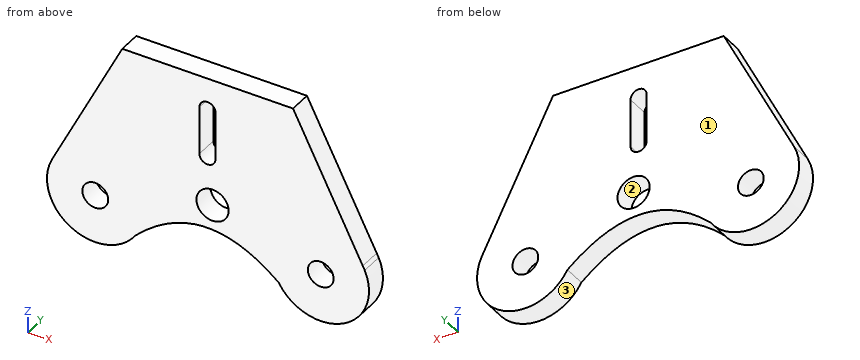
```python
from build123d import *

# Parameters (mm, degrees)
BOSS_EXTRUDE1_DEPTH = 8.89
CUT_EXTRUDE1_DEPTH  = 8.89
SKETCH3_R           = 5.08
CUT_EXTRUDE2_DEPTH  = 8.89
SKETCH4_R           = 5.08
CUT_EXTRUDE3_DEPTH  = 8.89
SKETCH5_R           = 6.35
CUT_EXTRUDE4_DEPTH  = 8.89


with BuildPart() as part:
    # Sketch1 → Boss-Extrude1 (new body)
    with BuildSketch(Plane(origin=(0, 0, 0), x_dir=(1, 0, 0), z_dir=(0, 1, 0))):
        with BuildLine():
            Line((-17.012597889, -8.571698377), (10.66270702, -63.5))
            Line((10.66270702, -63.5), (77.97270702, -63.5))
            Line((77.97270702, -63.5), (105.474181334, -9.391432964))
            Line((105.474181334, -9.391432964), (106.255653047, -7.853903954))
            ThreePointArc((106.255653047, -7.853903954), (97.513383696, 16.99153087), (72.305806006, 9.35602617))
            add(Edge.make_bspline(
                [(15.794561963, 10.650554558), (42.737740309, -15.557403772), (72.305806006, 9.35602617)],
                knots=[0, 0, 0, 1, 1, 1], degree=2))
            ThreePointArc((15.794561963, 10.650554558), (-9.630402632, 16.436479098), (-17.012597889, -8.571698377))
        make_face()
    extrude(amount=BOSS_EXTRUDE1_DEPTH)

    # Sketch2 → Cut-Extrude1 (cut)
    with BuildSketch(Plane(origin=(0, 8.89, 0), x_dir=(1, 0, 0), z_dir=(0, 1, 0))):
        with BuildLine():
            Line((47.406198559, -31.75), (47.406198559, -50.8))
            ThreePointArc((47.406198559, -50.8), (44.231198559, -53.975), (41.056198559, -50.8))
            Line((41.056198559, -50.8), (41.056198559, -31.75))
            ThreePointArc((41.056198559, -31.75), (44.231198559, -28.575), (47.406198559, -31.75))
        make_face()
    extrude(amount=-CUT_EXTRUDE1_DEPTH, mode=Mode.SUBTRACT)

    # Sketch3 → Cut-Extrude2 (cut)
    with BuildSketch(Plane(origin=(0, 8.89, 0), x_dir=(1, 0, 0), z_dir=(0, 1, 0))):
        with Locations(Location((0, 0, 0), (0, 0, 270))):
            Circle(SKETCH3_R)
    extrude(amount=-CUT_EXTRUDE2_DEPTH, mode=Mode.SUBTRACT)

    # Sketch4 → Cut-Extrude3 (cut)
    with BuildSketch(Plane(origin=(0, 8.89, 0), x_dir=(1, 0, 0), z_dir=(0, 1, 0))):
        with Locations(Location((88.9, 0, 0), (0, 0, 270))):
            Circle(SKETCH4_R)
    extrude(amount=-CUT_EXTRUDE3_DEPTH, mode=Mode.SUBTRACT)

    # Sketch5 → Cut-Extrude4 (cut)
    with BuildSketch(Plane(origin=(0, 8.89, 0), x_dir=(1, 0, 0), z_dir=(0, 1, 0))):
        with Locations(Location((46.230762454, -12.7, 0), (0, 0, 270))):
            Circle(SKETCH5_R)
    extrude(amount=-CUT_EXTRUDE4_DEPTH, mode=Mode.SUBTRACT)


solid = part.part
```
Part model, mm, in its own coordinate system. Face numbers are marked on the shaded views. Coordinates: 2 decimals unless noted, no trailing zeros. Loops run counter-clockwise (first coordinate to the right, second up) from the corner with the lowest first, then second, coordinate; pieces in that order, holes last. Notation, with made-up numbers: (30.25, -32.5) - (59.25, -32.5) arc R17 ccw to (59.25, -17.5) - close; hole circle Ø2 at (-22, 22). An arc over 180 degrees is marked (long way). Write item = value, one per line. Start each with the question number.
Item 1: Wall check: L1, parallel to X at y = 2, z = 0; L2, parallel to X at y = 7, z = -0.5; L3, parallel to X at y = 4.75, z = 12.7. Give the ranges that are in metal, low to high. Write a range as from..to.
Item 2: Cut at C-C, the plane x = 43. State how many separate pieces and enclosed holes the cut face has, and give its area (3 significant figures).
Item 3: Cut at B-B, the plane x = 86. Give the cut face in (y, z), and give its area (3 significant figures).
Item 4: Mould opens along Z. For the marked faces 1, 2 and 3 say: released by +Z, released by -Z, zero draft, split by the parting line, or undercut.
Item 5: Flat gauge pins, fed straight in: pin 1 Ø1 at (x, y) = (27, 7.5) entering from -Z; pin 2 Ø1 at (y, z) = (2, 6) entering from +X; pin 3 Ø1.5 at (x, y) = (28.5, 2) entering from -Z. Where does each tip first touch, or does it go through?
Item 6: Cut at A-A, the plane z = 12.7. Give the cut face in (x, y), and give its area (3 significant figures).
The answers:
q1.L1 = -19.05..-5.08, 5.08..31.05, 57.46..83.82, 93.98..107.95
q1.L2 = -19.04..-5.06, 5.06..29.94, 58.62..83.84, 93.96..107.94
q1.L3 = -14.93..39.88, 52.58..103.79
q2.separate_pieces = 3
q2.enclosed_holes = 0
q2.area = 221 mm2
q3.outline = (0, -18.83) - (8.89, -18.83) - (8.89, -4.17) - (0, -4.17) - close; (0, 4.17) - (8.89, 4.17) - (8.89, 47.71) - (0, 47.71) - close
q3.area = 517 mm2
q4.face_1 = zero draft
q4.face_2 = undercut
q4.face_3 = split by the parting line
q5.pin_1 = -2.32
q5.pin_2 = 107.14
q5.pin_3 = -1.61
q6.outline = (-14.93, 0) - (39.88, 0) - (39.88, 8.89) - (-14.93, 8.89) - close; (52.58, 0) - (103.79, 0) - (103.79, 8.89) - (52.58, 8.89) - close
q6.area = 943 mm2
